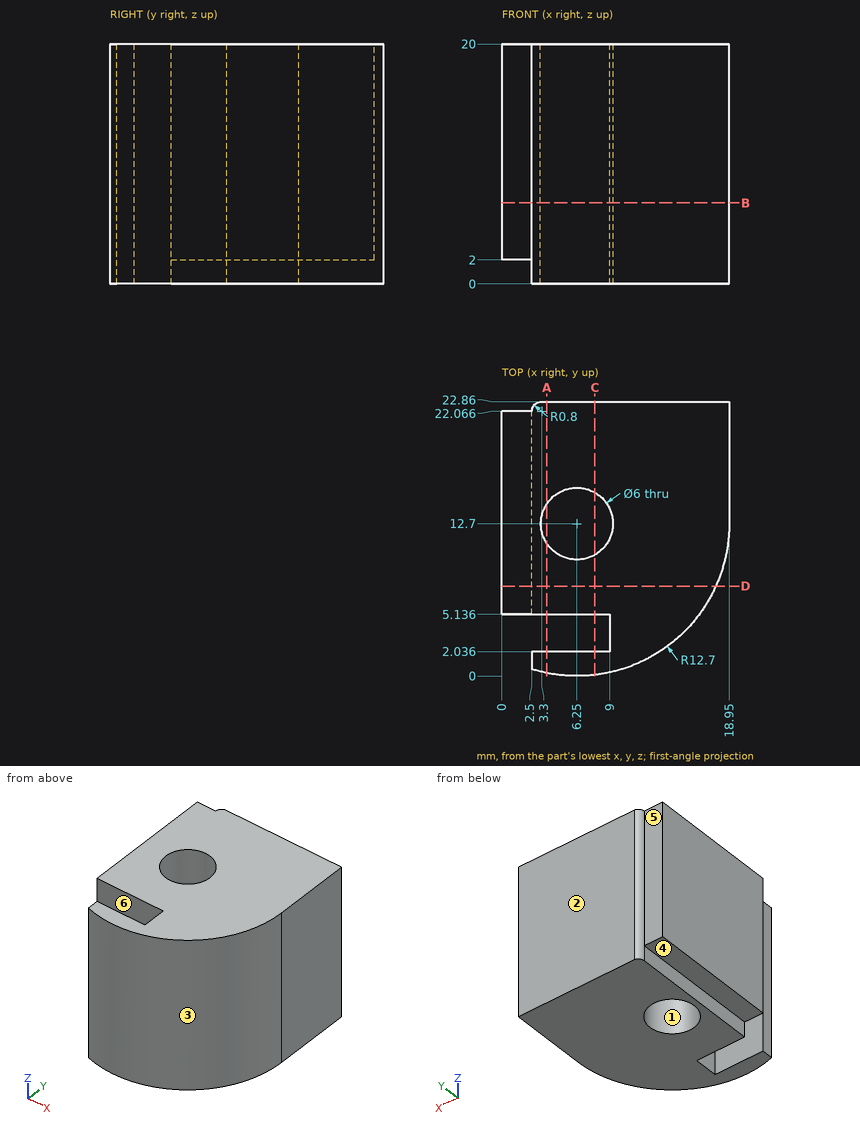
Source: three-view drawing plus pictorial views. Frame: mm from the lowest corner of the part. A direction names the side the tool comes from. Round coordinates to 2 decimals unless told otherwise and drop trailing zeros. Write each loop counter-clockwise with the first axis right and the second up, starting at its lowest first coordinate (ties: lowest second). Pieces come first, ordered by that corner, then holes. Notation, with made-up numbers: M -24,89 L 33,89 A22 ccw 33,121 Z; hole C 85,0.25 d4. An arc over 180 degrees is marked long. One line per item, written item: value. Start each with the question number.
Item 1: Pin query (flat end, axial travel): pin 1 (1.6 mm diameter, centred on y = 16.5, z = 0.5, fed in from -X); pin 2 (1.2 mm diameter, centred on x = 1, z = 10.5, fed in from +Y); pin 3 (2 mm diameter, centred on x = 1, y = 16.5, fed in from -Z). Return the tip coordinate at first contact, or that it passes through.
Item 2: Section query C-C (x = 7.75). Return the cut outline in (y, z).
Item 3: Section query B-B (z = 6.75). Return the cut outline in (x, y).
Item 4: Section query A-A (x = 3.75). Return the cut outline in (y, z).
Item 5: Ray query, L1, parallel to X at y = 12.7, z = 13.25; L2, parallel to Y at x = 5.75, z = 12.5; L3, parallel to Y at x = 8.25, z = 7.5 (1 decimal). Return the intervals inside material, ascending. Write a range as from..to.
Item 6: Mould query, pull axis Y, two halves, no side actions, for the marked faces 1, 2 and 3. Classes: pulls with the +Y half, pulls with the -Y half, needs draft (parallel to the pull), parting line crosses it, or undercut.
Item 7: Section query D-D (y = 7.5). Return the cut outline in (x, z), plus the area to 3 significant figures.
Item 8: Set-up query: the marked faces 4, 5 and 6. Return all of +Z, -Z, +X, -X, +Y, -Y with unobstructed straight access to the full face (end or side cutting, diameter ignored); none if empty.
Result set:
1. pin 1: stops at x = 2.5
1. pin 2: stops at y = 22.07
1. pin 3: stops at z = 2
2. outline: M 0.09,0 L 2.04,0 L 2.04,20 L 0.09,20 Z; M 5.14,0 L 10.1,0 L 10.1,20 L 5.14,20 Z; M 15.3,0 L 22.86,0 L 22.86,20 L 15.3,20 Z
3. outline: M 0,5.14 L 9,5.14 L 9,2.04 L 2.5,2.04 L 2.5,0.57 A12.7 ccw 18.95,12.7 L 18.95,22.86 L 3.2,22.86 A0.8 ccw 2.5,22.07 L 0,22.07 Z; hole C 6.25,12.7 d6
4. outline: M 0.25,0 L 2.04,0 L 2.04,20 L 0.25,20 Z; M 5.14,0 L 11.04,0 L 11.04,20 L 5.14,20 Z; M 14.36,0 L 22.86,0 L 22.86,20 L 14.36,20 Z
5. L1: x = 0..3.25, 9.25..18.95
5. L2: y = 0.01..2.04, 5.14..9.74, 15.66..22.86
5. L3: y = 0.2..2, 5.1..10.5, 14.9..22.9
6. face 1: undercut
6. face 2: pulls with the +Y half
6. face 3: pulls with the -Y half
7. outline: M 0,2 L 2.5,2 L 2.5,0 L 17.84,0 L 17.84,20 L 0,20 Z
7. area: 352 mm²
8. face 4: -Z, -X, +Y, -Y
8. face 5: +Z, -Z, -X, +Y
8. face 6: +Z, -Z, -X
